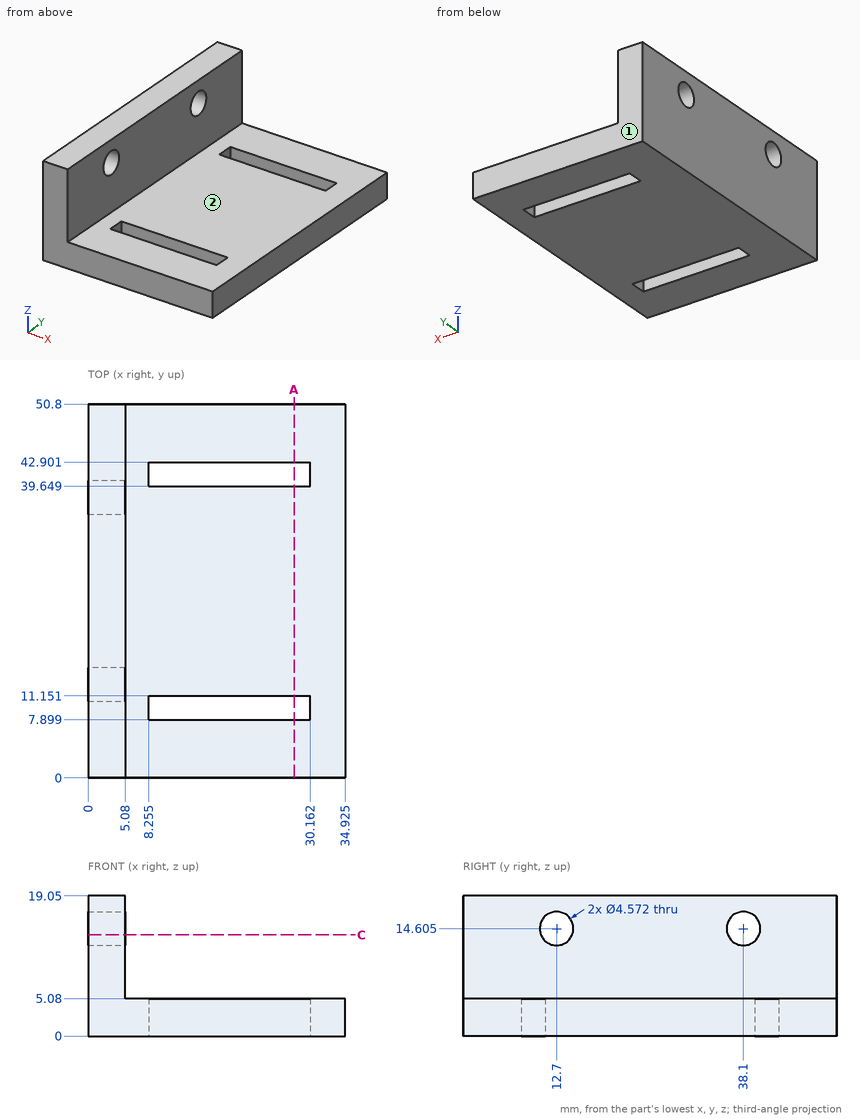
Source: three-view drawing plus pictorial views. Frame: mm from the lowest corner of the part. A direction names the side the tool comes from. Give positions to 0.01 mm unless a question says otherwise; leave off trailing zeros. Order: outer loops, then holes, each group sorted by start corner. A loop starts at its lowest first (then second) coordinate and runs counter-clockwise, first axis right, second up. Notation, with made-up numbers: (58.5, 12) - (113.5, 12) arc R33 cw to (113.5, 42) - close; hole circle Ø11 at (50, -35). An arc over 180 degrees is marked (long way). Answer as a JSON object with one key per item and string values. Group by question number.
Q1. Cut plane A-A, the plane x = 28. Output: boundary loops of the cut face in (y, z).
Q2. Line query: probe 1 along Y at (x, z) = (12, 1); probe 2 along Z at (x, y) = (3, 38); probe 3 along Z at (x, y) = (19.5, 48.5). Output: solid intervals per line, ascending.
Q3. Set-up query: the marked faces 1 and 2. Return all of +Z, -Z, +X, -X, +Y, -Y with unobstructed straight access to the full face (end or side cutting, diameter ignored); none if empty.
Q4. First-contact query: pin 1 Ø6 at (y, z) = (12.7, 14.605) entering from +X; pin 2 Ø2 at (x, y) = (21.5, 36) entering from +Z. Flat tips, straight axial feed; report the tip coordinate or a pass-through.
Q5. Cut plane C-C, the plane z = 13.75. Output: boundary loops of the cut face in (x, y), then the cut area to 3 significant figures.
Results:
{
 "1": {"outline": "(0, 0) - (7.9, 0) - (7.9, 5.08) - (0, 5.08) - close; (11.15, 0) - (39.65, 0) - (39.65, 5.08) - (11.15, 5.08) - close; (42.9, 0) - (50.8, 0) - (50.8, 5.08) - (42.9, 5.08) - close"},
 "2": {"probe 1": "0 to 7.9, 11.15 to 39.65, 42.9 to 50.8", "probe 2": "0 to 12.32, 16.89 to 19.05", "probe 3": "0 to 5.08"},
 "3": {"face 1": "+Z, -Z, +X, -X, +Y", "face 2": "+Z, +X, +Y, -Y"},
 "4": {"pin 1": "x = 5.08", "pin 2": "z = 5.08"},
 "5": {"outline": "(0, 0) - (5.08, 0) - (5.08, 10.58) - (0, 10.58) - close; (0, 14.82) - (5.08, 14.82) - (5.08, 35.98) - (0, 35.98) - close; (0, 40.22) - (5.08, 40.22) - (5.08, 50.8) - (0, 50.8) - close", "area": "215 mm^2"}
}
